Could you check a few things on this model? Use its own coordinates, in mm. A direction names the side the tool comes from. Give positions to 0.01 mm unless a question says otherwise; leave off trailing zeros. Loops run counter-clockwise (first coordinate to the right, second up) from the corner with the lowest first, then second, coordinate; pieces in that order, holes last. Notation, with made-up numbers: M -26,8.25 L 23,8.25 A10 cw 23,16.25 Z; hole C -37,53 d2. An arc over 180 degrees is marked long. Use a Markdown table: item, result. Add a question column.
1) Which directions (+Z, -Z, +X, -X, +Y, -Y) give clear straight access to the entire face, cutting with the end or side of a thin tool? Please do faces 1 (the flat face through (36, 36, 5)), 2 (the flat face through (36, -36, 5)), 3 (the flat face through (0, 0, 19.05)), 4 (the flat face through (-31, 31, 5)), 5 (the flat face through (-36, -36, 5)).
2) Will these pins go through, and if not, where does the flat tip stop? pin 1 Ø1 at (y, z) = (20, 9.5) entering from +X; pin 2 Ø10 at (y, z) = (21, 11.5) entering from -X; pin 3 Ø7.5 at (x, y) = (41.5, -11) entering from +Z.
3) Suppose I cut it at C-C on z = 17. List the corners of the cut face in (x, y) for me, and give its area (3 significant figures).
4) Suppose I cut it at D-D on x = -31. List the corners of the cut face in (y, z) for me, and give its area (3 significant figures).
5) If I drill on line 1 along Z through (x, y) = (35, -45); line 2 along X through (y, z) = (1, 14.75); line 3 along Y through (x, z) = (-6, 12.5), over which ranges is the centre line in solid material (lowest first)? Write a range as [from, to].
6) Suppose I cut it at A-A on y = -38. List the corners of the cut face in (x, z) for me.
```python
from build123d import *

# Parameters (mm, degrees)
F1_DEPTH = 5
F2_DEPTH = 12.7
F3_DEPTH = 19.05


with BuildPart() as f1:
    # F0 (on Top) → F1 (new body)
    with BuildSketch(Plane.XY):
        Polygon((50, 0), (50, 50), (0, 50), (25.0000000711, 24.9999999289), align=None)
        Polygon((-24.9999998008, 25.0000001992), (0, 50), (-50, 50), (-50, 0), align=None)
        Polygon((50, -50), (50, 0), (25.000000115, -24.999999885), (0, -50), align=None)
        with BuildLine():
            ThreePointArc((25.0000000711, 24.9999999289), (1.911e-07, 35.3553390593), (-24.9999998008, 25.0000001992))
            ThreePointArc((-24.9999998008, 25.0000001992), (-35.3553390593, 1.963e-07), (-25.0000000784, -24.9999999216))
            ThreePointArc((-25.0000000784, -24.9999999216), (2.59e-08, -35.3553390593), (25.000000115, -24.999999885))
            ThreePointArc((25.000000115, -24.999999885), (32.664074153, -13.5299024285), (35.3553390593, 0))
            ThreePointArc((35.3553390593, 0), (32.6640741411, 13.5299024572), (25.0000000711, 24.9999999289))
        make_face()
        with BuildLine():
            Line((25.0000000711, 24.9999999289), (0, 50))
            Line((0, 50), (-24.9999998008, 25.0000001992))
            ThreePointArc((-24.9999998008, 25.0000001992), (1.911e-07, 35.3553390593), (25.0000000711, 24.9999999289))
        make_face()
        with BuildLine():
            ThreePointArc((-25.0000000784, -24.9999999216), (-35.3553390593, 1.963e-07), (-24.9999998008, 25.0000001992))
            Line((-24.9999998008, 25.0000001992), (-50, 0))
            Line((-50, 0), (-25.0000000784, -24.9999999216))
        make_face()
        Polygon((-25.0000000784, -24.9999999216), (-50, 0), (-50, -50), (0, -50), align=None)
        with BuildLine():
            Line((25.000000115, -24.999999885), (50, 0))
            Line((50, 0), (25.0000000711, 24.9999999289))
            ThreePointArc((25.0000000711, 24.9999999289), (32.6640741411, 13.5299024572), (35.3553390593, 0))
            ThreePointArc((35.3553390593, 0), (32.664074153, -13.5299024285), (25.000000115, -24.999999885))
        make_face()
        with BuildLine():
            Line((0, -50), (25.000000115, -24.999999885))
            ThreePointArc((25.000000115, -24.999999885), (2.59e-08, -35.3553390593), (-25.0000000784, -24.9999999216))
            Line((-25.0000000784, -24.9999999216), (0, -50))
        make_face()
    extrude(amount=F1_DEPTH)

    # F0 (on Top) → F2 (join)
    with BuildSketch(Plane.XY):
        with BuildLine():
            ThreePointArc((-25.0000000784, -24.9999999216), (-35.3553390593, 1.963e-07), (-24.9999998008, 25.0000001992))
            Line((-24.9999998008, 25.0000001992), (-50, 0))
            Line((-50, 0), (-25.0000000784, -24.9999999216))
        make_face()
        with BuildLine():
            Line((25.000000115, -24.999999885), (50, 0))
            Line((50, 0), (25.0000000711, 24.9999999289))
            ThreePointArc((25.0000000711, 24.9999999289), (32.6640741411, 13.5299024572), (35.3553390593, 0))
            ThreePointArc((35.3553390593, 0), (32.664074153, -13.5299024285), (25.000000115, -24.999999885))
        make_face()
        with BuildLine():
            Line((0, -50), (25.000000115, -24.999999885))
            ThreePointArc((25.000000115, -24.999999885), (2.59e-08, -35.3553390593), (-25.0000000784, -24.9999999216))
            Line((-25.0000000784, -24.9999999216), (0, -50))
        make_face()
        with BuildLine():
            ThreePointArc((25.0000000711, 24.9999999289), (1.911e-07, 35.3553390593), (-24.9999998008, 25.0000001992))
            ThreePointArc((-24.9999998008, 25.0000001992), (-35.3553390593, 1.963e-07), (-25.0000000784, -24.9999999216))
            ThreePointArc((-25.0000000784, -24.9999999216), (2.59e-08, -35.3553390593), (25.000000115, -24.999999885))
            ThreePointArc((25.000000115, -24.999999885), (32.664074153, -13.5299024285), (35.3553390593, 0))
            ThreePointArc((35.3553390593, 0), (32.6640741411, 13.5299024572), (25.0000000711, 24.9999999289))
        make_face()
        with BuildLine():
            Line((25.0000000711, 24.9999999289), (0, 50))
            Line((0, 50), (-24.9999998008, 25.0000001992))
            ThreePointArc((-24.9999998008, 25.0000001992), (1.911e-07, 35.3553390593), (25.0000000711, 24.9999999289))
        make_face()
    extrude(amount=F2_DEPTH)

    # F0 (on Top) → F3 (join)
    with BuildSketch(Plane.XY):
        with BuildLine():
            ThreePointArc((25.0000000711, 24.9999999289), (1.911e-07, 35.3553390593), (-24.9999998008, 25.0000001992))
            ThreePointArc((-24.9999998008, 25.0000001992), (-35.3553390593, 1.963e-07), (-25.0000000784, -24.9999999216))
            ThreePointArc((-25.0000000784, -24.9999999216), (2.59e-08, -35.3553390593), (25.000000115, -24.999999885))
            ThreePointArc((25.000000115, -24.999999885), (32.664074153, -13.5299024285), (35.3553390593, 0))
            ThreePointArc((35.3553390593, 0), (32.6640741411, 13.5299024572), (25.0000000711, 24.9999999289))
        make_face()
    extrude(amount=F3_DEPTH)


solid = f1.part
```
Answer block:
| question | item | result |
|---|---|---|
| 1 | face 1 | +Z, +X, +Y |
| 1 | face 2 | +Z, +X, -Y |
| 1 | face 3 | +Z, +X, -X, +Y, -Y |
| 1 | face 4 | +Z, -X, +Y |
| 1 | face 5 | +Z, -X, -Y |
| 2 | pin 1 | stops at x = 30.5 |
| 2 | pin 2 | stops at x = -34 |
| 2 | pin 3 | stops at z = 12.7 |
| 3 | outline | C 0,0 d70.71 |
| 3 | area | 3,930 mm^2 |
| 4 | outline | M -50,0 L 50,0 L 50,5 L 19,5 L 19,12.7 L 17,12.7 L 17,19.05 L -17,19.05 L -17,12.7 L -19,12.7 L -19,5 L -50,5 Z |
| 4 | area | 1,010 mm^2 |
| 5 | line 1 | z = [0, 5] |
| 5 | line 2 | x = [-35.34, 35.34] |
| 5 | line 3 | y = [-44, 44] |
| 6 | outline | M -50,0 L 50,0 L 50,5 L 12,5 L 12,12.7 L -12,12.7 L -12,5 L -50,5 Z |
